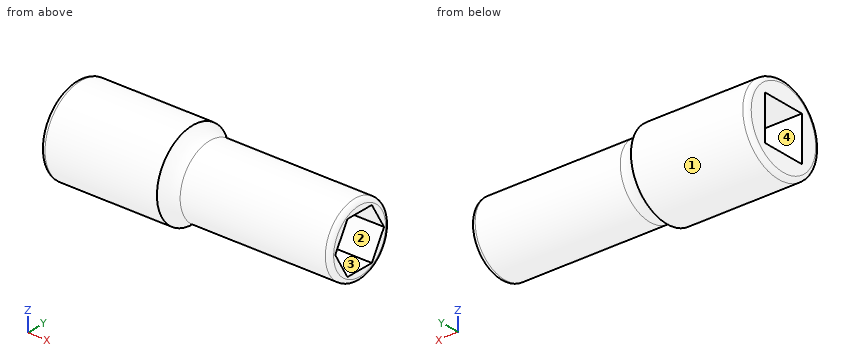
```python
from build123d import *

# Parameters (mm, degrees)
F0_R     = 9.5
F1_DEPTH = 31
F2_R     = 9.5
F2_R_2   = 7.845
F3_DEPTH = 36.5
F5_R     = 1
F7_DEPTH = 29
F8_W     = 9.7
F8_H     = 9.7
F9_DEPTH = 15


# Not quite as in the source:
# - a fillet or chamfer that OpenCascade refuses, or shapes differently, is made with other operations: its cross-section is extruded or revolved along the edge and cut away or added


with BuildPart() as f1:
    # F0 (on Right) → F1 (new body, symmetric)
    with BuildSketch(Plane.YZ):
        Circle(F0_R)
    extrude(amount=F1_DEPTH, both=True)

    # F2 (on face) → F3 (cut)
    with BuildSketch(Plane.YZ.offset(31)):
        Circle(F2_R)
        Circle(F2_R_2, mode=Mode.SUBTRACT)
    extrude(amount=-F3_DEPTH, mode=Mode.SUBTRACT)

    # F4: fillet of radius 5 on 1 edges, made by hand

    # F4_s1 → F4_t2 (revolve)
    with BuildSketch(Plane.XY):
        with BuildLine():
            ThreePointArc((-5.5, 9.5), (-3.8177725447, 8.2774514234), (-1.783687984, 7.845))
            Line((-1.783687984, 7.845), (-5.5, 7.845))
            Line((-5.5, 7.845), (-5.5, 9.5))
        make_face()
    revolve(axis=Axis((-5.5, 0, 0), (1, 0, 0)))

    # F5
    f5_edges = [f1.edges().sort_by_distance(p)[0] for p in [
        (31, -7.845, 0),
        (-31, -9.5, 0),
    ]]
    fillet(f5_edges, radius=F5_R)

    # F6 (on face) → F7 (cut)
    with BuildSketch(Plane.YZ.offset(31)):
        Polygon((3.212954248, 5.565), (-3.212954248, 5.565), (-6.4259084961, 0), (-3.212954248, -5.565), (3.212954248, -5.565), (6.4259084961, 0), align=None)
    extrude(amount=-F7_DEPTH, mode=Mode.SUBTRACT)

    # F8 (on face) → F9 (cut)
    with BuildSketch(Plane(origin=(-31, 0, 0), x_dir=(0, -1, 0), z_dir=(-1, 0, 0))):
        Rectangle(F8_W, F8_H)
    extrude(amount=-F9_DEPTH, mode=Mode.SUBTRACT)


solid = f1.part
```
Build history of the part. All positions in model axes, mm. Face numbers are marked on the shaded views. A direction names the side the tool comes from. Give positions to 0.01 mm unless a question says otherwise; leave off trailing zeros. Loops run counter-clockwise (first coordinate to the right, second up) from the corner with the lowest first, then second, coordinate; pieces in that order, holes last. Notation, with made-up numbers: (-2.75, -21) - (34.25, -21) arc R15 cw to (34.25, -15) - close; hole circle Ø2 at (-32, 46). An arc over 180 degrees is marked (long way). Use a Markdown table: item, result.
(1) Pull direction Z, two halves, no side cores. Call the marked faces 1 and 2: +Z half, -Z half, draft (parallel to the pull), parting line (faces both ways), or undercut.
Taken from the geometry:
| item | result |
|---|---|
| face 1 | parting line |
| face 2 | undercut |
(2) Which spindle directions (+Z, -Z, +X, -X, +Y, -Y) get a long thin tool onto all of the face, cutting with end or side? Do the marked faces 3 and 4. Say none if no direction does.
Taken from the geometry:
| item | result |
|---|---|
| face 3 | +X |
| face 4 | -X |
(3) Wall check: line 1 along X through (y, z) = (-0.5, 3); line 2 along Z through (x, y) = (-21, 0.25); line 3 along Y through (x, z) = (12, 2). Give the ranges that are in metal, low to high.
Taken from the geometry:
| item | result |
|---|---|
| line 1 | -16 to 2 |
| line 2 | -9.5 to -4.85, 4.85 to 9.5 |
| line 3 | -7.59 to -5.27, 5.27 to 7.59 |
(4) Drop flat-ended pins along their axis: pin 1 Ø4 at (y, z) = (-1.5, 1.5) entering from -X; pin 2 Ø3 at (x, y) = (16.5, -5) entering from +Z; pin 3 Ø2 at (x, y) = (16.5, 3) entering from -Z. Give the stop position or say it passes through.
Taken from the geometry:
| item | result |
|---|---|
| pin 1 | x = -16 |
| pin 2 | z = 7.02 |
| pin 3 | z = -7.59 |
(5) Band-saw the part on B-B (y = 0). Give the cut face in (x, z) (3 decimals), and give its area (3 significant figures).
Taken from the geometry:
| item | result |
|---|---|
| outline | (-31, -8.5) arc R1 ccw to (-30, -9.5) - (-5.5, -9.5) arc R5 cw to (-1.784, -7.845) - (30, -7.845) arc R1 ccw to (31, -6.845) - (31, -5.565) - (2, -5.565) - (2, 5.565) - (31, 5.565) - (31, 6.845) arc R1 ccw to (30, 7.845) - (-1.784, 7.845) arc R5 cw to (-5.5, 9.5) - (-30, 9.5) arc R1 ccw to (-31, 8.5) - (-31, 4.85) - (-16, 4.85) - (-16, -4.85) - (-31, -4.85) - close |
| area | 592 mm2 |
(6) Band-saw the part on C-C (x = 1). Give the cut face in (y, z) (3 decimals), and give its area (3 significant figures).
Taken from the geometry:
| item | result |
|---|---|
| outline | circle Ø15.69 at (0, 0) |
| area | 193 mm2 |
(7) Band-saw the part on A-A (x = 14.5). Give the cut face in (y, z) (3 decimals), and give its area (3 significant figures).
Taken from the geometry:
| item | result |
|---|---|
| outline | circle Ø15.69 at (0, 0); hole (-6.426, 0) - (-3.213, -5.565) - (3.213, -5.565) - (6.426, 0) - (3.213, 5.565) - (-3.213, 5.565) - close |
| area | 86.1 mm2 |
